Model file for the job. Use its own axes, mm. Coordinates: 2 decimals unless noted, no trailing zeros. Write each loop counter-clockwise with the first axis right and the second up, starting at its lowest first coordinate (ties: lowest second). Pieces come first, ordered by that corner, then holes. Notation, with made-up numbers: M 39.5,-1.5 L 97.5,-1.5 A20 cw 97.5,15.5 Z; hole C 4.5,46 d2. An arc over 180 degrees is marked long. One line per question, with ' | ' between items. Start each with the question number.
(1) Flat gauge pins, fed straight in: pin 1 Ø1.5 at (x, y) = (-99, 1) entering from -Z; pin 2 Ø2 at (x, z) = (-215, 12.5) entering from +Y; pin 3 Ø1.9 at (x, y) = (189.5, 2) entering from +Z; pin 4 Ø3 at (y, z) = (2.5, -58.5) entering from -X. Where does each tip first touch, or does it go through?
(2) Wall check: probe 1 along X at (y, z) = (2, 12.5); probe 2 along X at (y, z) = (3.75, 62.5); probe 3 along Z at (x, y) = (-215, 2). Give the ranges that are in metal, low to high.
(3) Cut at B-B (y = 2). Count the separate pieces of the cut face and the enclosed holes in it, plus the area to 3 significant figures.
(4) Cut at A-A (z = 42). Write the cut outline in (x, y).
(5) Cut at C-C (x = 118). Write the cut outline in (y, z).
from build123d import *

# Parameters (mm, degrees)
BOSS_EXTRUDE2_DEPTH       = 6.35
SKETCH2_R                 = 1.75
CUT_EXTRUDE1_DEPTH        = 6.35
LPATTERN1_COUNT           = 2
LPATTERN1_PITCH           = 25
LPATTERN2_COUNT           = 2
LPATTERN2_PITCH           = 25
LPATTERN2_COPY_1_SKETCH_R = 1.75
LPATTERN2_COPY_1_DEPTH    = 6.35
FILLET1_R                 = 10
SKETCH3_R                 = 1.75
CUT_EXTRUDE2_DEPTH        = 7.35
SKETCH5_R                 = 1.75
CUT_EXTRUDE3_DEPTH        = 7.35
LPATTERN3_COUNT           = 2
LPATTERN3_PITCH           = 405
LPATTERN3_COPY_1_SKETCH_R = 1.75
LPATTERN3_COPY_1_DEPTH    = 6.35
LPATTERN3_COPY_2_SKETCH_R = 1.75
LPATTERN3_COPY_2_DEPTH    = 6.35
LPATTERN3_COPY_3_SKETCH_R = 1.75
LPATTERN3_COPY_3_DEPTH    = 6.35


with BuildPart() as part:
    # Sketch1 → Boss-Extrude2 (new body)
    with BuildSketch(Plane(origin=(0, 0, 0), x_dir=(1, 0, 0), z_dir=(0, 1, 0))):
        Polygon((-240, 37.5), (150, 37.5), (150, 87.5), (180, 87.5), (180, 37.5), (210, 37.5), (210, 87.5), (240, 87.5), (240, -87.5), (210, -87.5), (210, -37.5), (180, -37.5), (180, -87.5), (150, -87.5), (150, -37.5), (-240, -37.5), align=None)
    extrude(amount=BOSS_EXTRUDE2_DEPTH)

    # Sketch2 → Cut-Extrude1 (cut)
    with BuildSketch(Plane(origin=(0, 6.35, 0), x_dir=(1, 0, 0), z_dir=(0, 1, 0))):
        with Locations((190, 12.5)):
            Circle(SKETCH2_R)
    cut_extrude1 = extrude(amount=-CUT_EXTRUDE1_DEPTH, mode=Mode.SUBTRACT)

    # LPattern1: Cut-Extrude1 ×2
    with Locations(*[(i * LPATTERN1_PITCH, 0, 0) for i in range(1, LPATTERN1_COUNT)]):
        add(cut_extrude1, mode=Mode.SUBTRACT)

    # LPattern2: Cut-Extrude1 ×2
    with Locations(*[(0, 0, i * LPATTERN2_PITCH) for i in range(1, LPATTERN2_COUNT)]):
        add(cut_extrude1, mode=Mode.SUBTRACT)

    # LPattern2 copy 1 sketch → LPattern2 copy 1 (cut)
    with BuildSketch(Plane(origin=(25, 6.35, 25), x_dir=(1, 0, 0), z_dir=(0, 1, 0))):
        with Locations((190, 12.5)):
            Circle(LPATTERN2_COPY_1_SKETCH_R)
    extrude(amount=-LPATTERN2_COPY_1_DEPTH, mode=Mode.SUBTRACT)

    # Fillet1
    fillet1_edges = [part.edges().sort_by_distance(p)[0] for p in [
        (-240, 3.175, -37.5),
        (150, 3.175, -87.5),
        (180, 3.175, -87.5),
        (210, 3.175, -87.5),
        (240, 3.175, -87.5),
        (240, 3.175, 87.5),
        (210, 3.175, 87.5),
        (180, 3.175, 87.5),
        (150, 3.175, 87.5),
        (-240, 3.175, 37.5),
    ]]
    fillet(fillet1_edges, radius=FILLET1_R)

    # Sketch3 → Cut-Extrude2 (cut, through all)
    with BuildSketch(Plane(origin=(0, 6.35, 0), x_dir=(1, 0, 0), z_dir=(0, 1, 0))):
        with Locations((224.12, 67.5)):
            Circle(SKETCH3_R)
        with Locations((224.12, -67.5)):
            Circle(SKETCH3_R)
    extrude(amount=-CUT_EXTRUDE2_DEPTH, mode=Mode.SUBTRACT)

    # Sketch5 → Cut-Extrude3 (cut, through all)
    with BuildSketch(Plane(origin=(0, 6.35, 0), x_dir=(1, 0, 0), z_dir=(0, 1, 0))):
        with Locations((165, 62.5)):
            Circle(SKETCH5_R)
        with Locations((165, -62.5)):
            Circle(SKETCH5_R)
    extrude(amount=-CUT_EXTRUDE3_DEPTH, mode=Mode.SUBTRACT)

    # LPattern3: Cut-Extrude1 ×2
    with Locations(*[(-i * LPATTERN3_PITCH, 0, 0) for i in range(1, LPATTERN3_COUNT)]):
        add(cut_extrude1, mode=Mode.SUBTRACT)

    # LPattern3 copy 1 sketch → LPattern3 copy 1 (cut)
    with BuildSketch(Plane(origin=(-405, 6.35, 25), x_dir=(1, 0, 0), z_dir=(0, 1, 0))):
        with Locations((190, 12.5)):
            Circle(LPATTERN3_COPY_1_SKETCH_R)
    extrude(amount=-LPATTERN3_COPY_1_DEPTH, mode=Mode.SUBTRACT)

    # LPattern3 copy 2 sketch → LPattern3 copy 2 (cut)
    with BuildSketch(Plane(origin=(-380, 6.35, 25), x_dir=(1, 0, 0), z_dir=(0, 1, 0))):
        with Locations((190, 12.5)):
            Circle(LPATTERN3_COPY_2_SKETCH_R)
    extrude(amount=-LPATTERN3_COPY_2_DEPTH, mode=Mode.SUBTRACT)

    # LPattern3 copy 3 sketch → LPattern3 copy 3 (cut)
    with BuildSketch(Plane(origin=(-380, 6.35, 0), x_dir=(1, 0, 0), z_dir=(0, 1, 0))):
        with Locations((190, 12.5)):
            Circle(LPATTERN3_COPY_3_SKETCH_R)
    extrude(amount=-LPATTERN3_COPY_3_DEPTH, mode=Mode.SUBTRACT)


solid = part.part
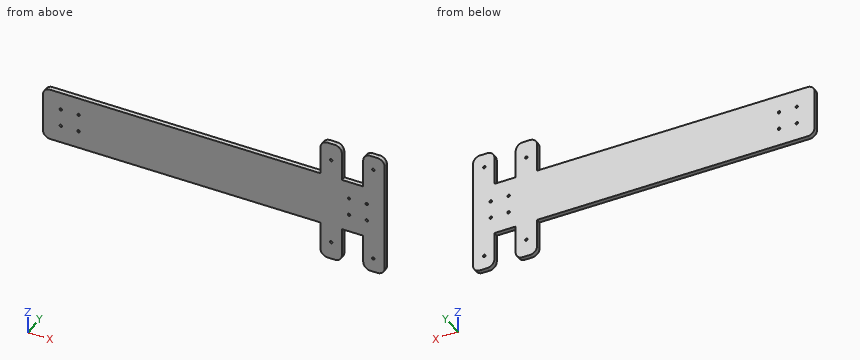
Filled in:
1) pin 1: z = -37.5 | pin 2: through | pin 3: z = 37.5 | pin 4: x = 150
2) probe 1: -240 to -216.75, -213.25 to -191.75, -188.25 to 188.25, 191.75 to 213.25, 216.75 to 240 | probe 2: 150 to 163.25, 166.75 to 180, 210 to 240 | probe 3: -37.5 to -14.25, -10.75 to 10.75, 14.25 to 37.5
3) separate pieces: 1 | enclosed holes: 12 | area: 41,700 mm²
4) outline: M 150,0 L 180,0 L 180,6.35 L 150,6.35 Z; M 210,0 L 240,0 L 240,6.35 L 210,6.35 Z
5) outline: M 0,-37.5 L 6.35,-37.5 L 6.35,37.5 L 0,37.5 Z
